Drawing for the job (mm, zero at the part's lowest x, y, z). A direction names the side the tool comes from. Give positions to 0.01 mm unless a question says otherwise; leave off trailing zeros. Loops run counter-clockwise (first coordinate to the right, second up) from the corner with the lowest first, then second, coordinate; pieces in that order, holes last.
1) 3-axis set-ups, long thin cutter, end or side, ignore diameter. For the marked faces 1 and 2: which of +Z, -Z, +X, -X, +Y, -Y reach the whole face in a straight line?
2) Flat gauge pins, fed straight in: P1, Ø1.5, axis at y = 8, z = 13, coming from the +X side; P2, Ø6, axis at x = 5.5, z = 6.5, coming from the +Y side; P3, Ø4, axis at y = 12, z = 27.5, coming from the +X side. Where does each tip first touch, or does it go through?
3) Wall check: line 1 (Z direction, x = 8.75, y = 14.25); line 2 (Y direction, x = 8.75, z = 17); line 3 (Y direction, x = 5, z = 30.5). Give the ranges that are in metal, low to high.
4) Band-saw the part on A-A on x = 9. List the corners of the cut face in (y, z).
5) Band-saw the part on C-C on z = 17. List the corners of the cut face in (x, y).
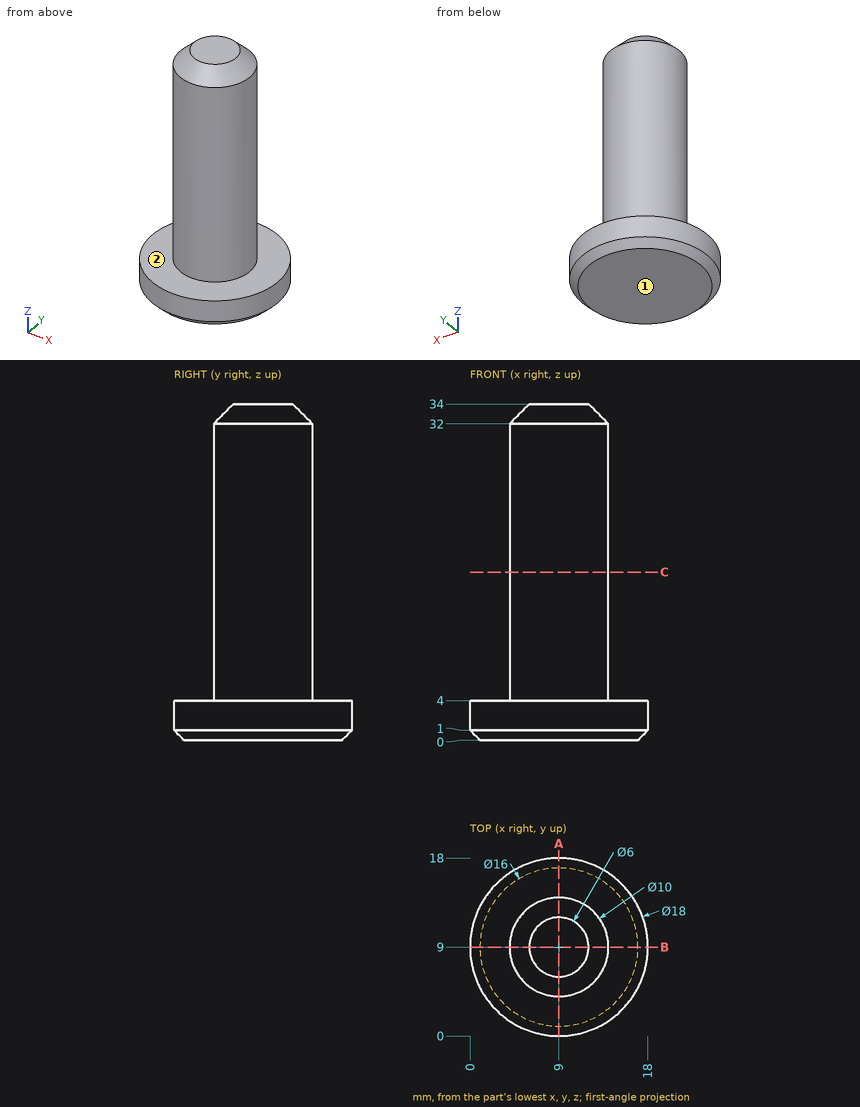
Findings below:
1. face 1: -Z, +X, -X, +Y, -Y
1. face 2: +Z
2. P1: stops at x = 13.99
2. P2: stops at y = 17.81
2. P3: stops at x = 13.9
3. line 1: z = 0 to 4
3. line 2: y = 4.01 to 13.99
3. line 3: y = 6 to 12
4. outline: (0, 1) - (1, 0) - (17, 0) - (18, 1) - (18, 4) - (14, 4) - (14, 32) - (12, 34) - (6, 34) - (4, 32) - (4, 4) - (0, 4) - close
5. outline: circle Ø10 at (9, 9)
